Work out the finished part from the listing and answer in its coordinate system (mm). A direction names the side the tool comes from. Coordinates: 2 decimals unless noted, no trailing zeros. Order: outer loops, then holes, each group sorted by start corner. A loop starts at its lowest first (then second) coordinate and runs counter-clockwise, first axis right, second up. Notation, with made-up numbers: (12, 4) -> (28, 4) arc R29 ccw to (28, 35) -> close; hole circle Ø3 at (0.25, 33). An arc over 180 degrees is marked (long way). Write item = value, one per line. Start each with the question number.
Q1. Straight lines are drawn through the part: L1, parallel to Z at x = 33.5, y = -9; L2, parallel to Y at x = 14, z = 10; L3, parallel to X at y = 11.5, z = 2. For each, find the intervals that lie inside material, in ascending order. Write a range as from..to.
Q2. Flat-ended cylindrical pins translate along their axes: pin 1 (10 mm diameter, centred on x = -28, z = 15.5, fed in from +Y); pin 2 (3 mm diameter, centred on x = -20.5, y = 27.5, fed in from -Z); pin 3 (3 mm diameter, centred on x = -2, z = 1, fed in from +Y). Find the tip coordinate at first contact, or state that the pin passes through.
Q3. The part is cut by section D-D, the plane z = -3. Determine the outline of the cut face in (x, y).
Q4. For a pull along Z with two mould halves and no side action, classify faces 1 (the flat face through (-5, 9.3, -37.95)), 2 (the flat face through (-1, 1, 27.6)), 3 (the flat face through (0, 0, -44.85)), 4 (the cylindrical face through (-8.227, -37.048, 13.607)) as +Z half, -Z half, draft (parallel to the pull), parting line (faces both ways), or undercut.
Q5. The part is cut by section A-A, the plane y = 0. Determine the outline of the cut face in (x, z).
Q6. The part is cut by section C-C, the plane z = 20.5. Determine the outline of the cut face in (x, y), plus the area to 3 significant figures.
Q7. Which of the six approach directions +Z, -Z, +X, -X, +Y, -Y give full straight-line access (tool end or side, diameter ignored) to faces 5 (the cylindrical face through (9.87, -3.11, -18.71)), 6 (the cylindrical face through (10.17, 9.33, -41.35))?
```python
from build123d import *

# Parameters (mm, degrees)
SKETCH_1_R      = 110
EXTRUDE_1_DEPTH = 80
SKETCH_2_R      = 30
EXTRUDE_2_DEPTH = 110
SKETCH_3_R      = 40
EXTRUDE_3_DEPTH = 20
SCALE_1_SCALE   = 0.345


with BuildPart() as part:
    # 草图1 → 凸台-拉伸1 (new body)
    with BuildSketch(Plane.XY):
        Circle(SKETCH_1_R)
    extrude(amount=EXTRUDE_1_DEPTH)

    # 草图2 → 凸台-拉伸2 (add)
    with BuildSketch(Plane(origin=(0, 0, 0), x_dir=(-1, 0, 0), z_dir=(0, 0, -1))):
        with Locations(Location((0, 0, 0), (0, 0, 180))):
            Circle(SKETCH_2_R)
    extrude(amount=EXTRUDE_2_DEPTH)

    # 草图3 → 凸台-拉伸3 (add)
    with BuildSketch(Plane(origin=(0, 0, -110), x_dir=(-1, 0, 0), z_dir=(0, 0, -1))):
        Circle(SKETCH_3_R)
    extrude(amount=EXTRUDE_3_DEPTH)


with BuildPart() as part_1:
    # 缩放比例1: scaled about (0, 0, 0)
    add(part.part.scale(SCALE_1_SCALE))


solid = part_1.part
```
Model answer:
q1.L1 = 0..27.6
q1.L2 = -35.27..35.27
q1.L3 = -36.17..36.17
q2.pin_1 = 30.19
q2.pin_2 = 0
q2.pin_3 = 37.95
q3.outline = circle Ø20.7 at (0, 0)
q4.face_1 = undercut
q4.face_2 = +Z half
q4.face_3 = -Z half
q4.face_4 = draft
q5.outline = (-37.95, 0) -> (-10.35, 0) -> (-10.35, -37.95) -> (-13.8, -37.95) -> (-13.8, -44.85) -> (13.8, -44.85) -> (13.8, -37.95) -> (10.35, -37.95) -> (10.35, 0) -> (37.95, 0) -> (37.95, 27.6) -> (-37.95, 27.6) -> close
q6.outline = circle Ø75.9 at (0, 0)
q6.area = 4,520 mm2
q7.face_5 = none
q7.face_6 = -Z
